Verification items for the finished model (mm, model axes). A direction names the side the tool comes from. Round coordinates to 2 decimals unless told otherwise and drop trailing zeros. Write each loop counter-clockwise with the first axis right and the second up, starting at its lowest first coordinate (ties: lowest second). Pieces come first, ordered by that corner, then holes. Notation, with made-up numbers: M -33.75,48 L 9.25,48 A35 cw 9.25,82 Z; hole C 71,-8.5 d10. An arc over 180 degrees is marked long. Answer in a Markdown table with one row per item. Add a question column.
1. Set-up check for faces 5 (the flat face through (25, 75, -37.5)), 6 (the flat face through (25, 75, -46.015)), 7 (the cylindrical face through (5.505, 6.451, -42.813)): record each of +Z, -Z, +X, -X, +Y, -Y from which the full face is reachable in a straight line by a thin tool's end or side.
2. Material ranges on probe 1 along X at (y, z) = (75, -40.5); probe 2 along Y at (x, z) = (35, -39); probe 3 along Z at (x, y) = (5, 7), recorded low to high.
3. Go/stop test with flat-tipped pins: pin 1 Ø2 at (x, y) = (16.5, 30) entering from -Z; pin 2 Ø2.5 at (x, y) = (35, 75) entering from -Z; pin 3 Ø4 at (x, y) = (42.5, 54) entering from -Z; pin 4 Ø1 at (x, z) = (43.5, -19.5) entering from -Y. Record where each tip stops, or that it passes through.
4. Sectioned sample at A-A on y = 75. Record the cut outline in (x, z).
5. Draft check along X on faces 1 (the flat face through (50, 42, -19)), 2 (the flat face through (25, 0, -44)), 3 (the flat face through (42.76, 1.48, -41.69)), 4 (the flat face through (2.669, 1, -6)). Enter one of: pulls with the +X half, pulls with the -X half, needs draft (parallel to the pull), parting line crosses it, or undercut.
6. Sectioned sample at B-B on z = -44.3. Record the cut outline in (x, y).
7. Sectioned sample at C-C on x = 34. Count the separate pieces of the cut face and the enclosed holes in it, plus the area to 3 significant figures.
Autodesk Inventor part; units mm, degrees
ref_plane "YZ Plane" through (0, 0, 0) normal (1, 0, 0) x (0, 1, 0)
ref_plane "XZ Plane" through (0, 0, 0) normal (0, 1, 0) x (-1, 0, 0)
ref_plane "XY Plane" through (0, 0, 0) normal (0, 0, 1) x (1, 0, 0)
sketch "Sketch1" plane through (0, 0, 0) normal (1, 0, 0) x (0, 1, 0)
  ellipse E0 centre (0, -25) end of major axis (45, -25) minor radius 12.5 (0, -37.5) -> (0, -12.5) ccw
  ellipse E1 centre (0, -25) end of major axis (120, -25) minor radius 25 (0, -50) -> (0, 0) ccw
  line L0 (65, -3.9852) -> (65, -46.0148)
  line L1 (0, -37.5) -> (0, -50)
  line L2 (0, -12.5) -> (0, 0)
  point P0 (0, -43.75)
  point P1 (0, -6.25)
  dimension "d23" = 45
  dimension "d25" = 120
  dimension "d18" = 50
  dimension "d22" = 25
  dimension "d24" = 65
extrude "Extrusion1" add sketch "Sketch1" along normal blind 50 contours E0 L2 E1 L0 L1
sketch "Sketch3" plane through (0, 65, -3.9852) normal (0, 1, 0) x (1, 0, 0)
  line L0 (0, 42.0297) -> (0, 0)
  line L1 (0, 0) -> (50, 0)
  line L2 (50, 42.0297) -> (50, 0)
  line L3 (0, 42.0297) -> (50, 42.0297)
  line L4 (0, 33.5148) -> (0, 8.5148)
  line L5 (50, 0) -> (0, 0)
  line L6 (0, 0) -> (0, 8.5148)
  line L7 (0, 8.5148) -> (50, 8.5148)
  line L8 (50, 8.5148) -> (50, 0)
  line L9 (0, 42.0297) -> (50, 42.0297)
  line L10 (50, 42.0297) -> (50, 33.5148)
  line L11 (50, 33.5148) -> (0, 33.5148)
  line L12 (0, 33.5148) -> (0, 42.0297)
  point P0 (0, -3.9852)
  point P1 (0, 33.5148)
  dimension "d26" = 25
  dimension "d27" = 8.5148
  dimension "d28" = 8.5148
extrude "Extrusion3" add sketch "Sketch3" along normal blind 20 contours L3 L2 L11 L0 | L7 L2 L1 L0
sketch "Sketch4" plane through (50, 65, -46.0148) normal (0, 0, -1) x (-1, 0, 0)
  line L0 (50, 0) -> (0, 0)
  line L1 (50, 0) -> (50, 20)
  line L2 (0, 20) -> (50, 20)
  line L3 (0, 0) -> (0, 20)
  line L4 (0, 0) -> (0, 20)
  line L5 (0, 10) -> (50, 10)
  circle A0 centre (15, 10) radius 2.25
  circle A1 centre (35, 10) radius 2.25
  point P0 (50, -65)
  dimension "d31" = 4.5
  dimension "d32" = 4.5
  dimension "d33" = 20
  dimension "d34" = 15
  dimension "d35" = 15
extrude "Extrusion4" cut sketch "Sketch4" against normal through all contours A1 L5 | L5 A1 | A0 L5 | L5 A0
sketch "Sketch5" plane through (0, 0, -12.5) normal (0, -1, 0) x (1, 0, 0)
  line L0 (0, 12.5) -> (0, 0)
  line L1 (0, 0) -> (50, 0)
  line L2 (50, 12.5) -> (50, 0)
  line L3 (0, 12.5) -> (50, 12.5)
  line L4 (0, -25) -> (0, -37.5)
  line L5 (0, -37.5) -> (50, -37.5)
  line L6 (50, -25) -> (50, -37.5)
  line L7 (0, -25) -> (50, -25)
  line L8 (50, 8.5148) -> (50, 12.5)
  line L9 (0, -25) -> (0, -37.5)
  line L10 (50, 12.5) -> (0, -37.5)
  line L11 (5.7, 6.8) -> (44.3, 6.8)
  line L12 (44.3, 6.8) -> (44.3, -31.8)
  line L13 (44.3, -31.8) -> (5.7, -31.8)
  line L14 (5.7, -31.8) -> (5.7, 6.8)
  line L15 (5.7, 6.8) -> (44.3, -31.8) construction
  line L16 (44.3, 6.8) -> (5.7, -31.8) construction
  line L17 (44.3, 3.3) -> (41.2689, 5.05)
  line L18 (41.2689, 5.05) -> (41.2689, 8.55)
  line L19 (41.2689, 8.55) -> (44.3, 10.3)
  line L20 (44.3, 10.3) -> (47.3311, 8.55)
  line L21 (47.3311, 8.55) -> (47.3311, 5.05)
  line L22 (47.3311, 5.05) -> (44.3, 3.3)
  line L23 (41.2689, -33.55) -> (41.2689, -30.05)
  line L24 (41.2689, -30.05) -> (44.3, -28.3)
  line L25 (44.3, -28.3) -> (47.3311, -30.05)
  line L26 (47.3311, -30.05) -> (47.3311, -33.55)
  line L27 (47.3311, -33.55) -> (44.3, -35.3)
  line L28 (44.3, -35.3) -> (41.2689, -33.55)
  line L29 (8.7311, -30.05) -> (8.7311, -33.55)
  line L30 (8.7311, -33.55) -> (5.7, -35.3)
  line L31 (5.7, -35.3) -> (2.6689, -33.55)
  line L32 (2.6689, -33.55) -> (2.6689, -30.05)
  line L33 (2.6689, -30.05) -> (5.7, -28.3)
  line L34 (5.7, -28.3) -> (8.7311, -30.05)
  line L35 (8.7311, 8.55) -> (8.7311, 5.05)
  line L36 (8.7311, 5.05) -> (5.7, 3.3)
  line L37 (5.7, 3.3) -> (2.6689, 5.05)
  line L38 (2.6689, 5.05) -> (2.6689, 8.55)
  line L39 (2.6689, 8.55) -> (5.7, 10.3)
  line L40 (5.7, 10.3) -> (8.7311, 8.55)
  point P0 (25, -12.5)
  dimension "d38" = 38.6
  dimension "d39" = 38.6
  dimension "d40" = 7
  dimension "d41" = 7
  dimension "d42" = 7
  dimension "d43" = 7
extrude "Extrusion5" cut sketch "Sketch5" against normal blind 3 contours L20 L21 L22 L12 L10 | L10 L11 L18 L19 L20 | L37 L38 L39 L40 L35 L11 L14 | L14 L11 L35 L36 | L12 L17 L10 | L10 L17 L18 L11 | L34 L10 L14 | L14 L10 L31 L32 L33 | L34 L29 L13 L10 | L13 L29 L30 L31 L10 | L25 L26 L27 L28 L23 L13 L12 | L12 L13 L23 L24
sketch "Sketch6" plane through (0, 0, -12.5) normal (0, -1, 0) x (1, 0, 0)
  line L0 (44.3, 10.3) -> (47.3311, 8.55)
  line L1 (41.2689, 8.55) -> (44.3, 10.3)
  line L2 (41.2689, 5.05) -> (41.2689, 8.55)
  line L3 (44.3, 3.3) -> (41.2689, 5.05)
  line L4 (47.3311, 5.05) -> (44.3, 3.3)
  line L5 (47.3311, 8.55) -> (47.3311, 5.05)
  line L6 (47.3311, -33.55) -> (44.3, -35.3)
  line L7 (47.3311, -30.05) -> (47.3311, -33.55)
  line L8 (44.3, -28.3) -> (47.3311, -30.05)
  line L9 (41.2689, -30.05) -> (44.3, -28.3)
  line L10 (41.2689, -33.55) -> (41.2689, -30.05)
  line L11 (44.3, -35.3) -> (41.2689, -33.55)
  line L12 (5.7, -35.3) -> (2.6689, -33.55)
  line L13 (8.7311, -33.55) -> (5.7, -35.3)
  line L14 (8.7311, -30.05) -> (8.7311, -33.55)
  line L15 (5.7, -28.3) -> (8.7311, -30.05)
  line L16 (2.6689, -30.05) -> (5.7, -28.3)
  line L17 (2.6689, -33.55) -> (2.6689, -30.05)
  line L18 (2.6689, 8.55) -> (5.7, 10.3)
  line L19 (2.6689, 5.05) -> (2.6689, 8.55)
  line L20 (5.7, 3.3) -> (2.6689, 5.05)
  line L21 (8.7311, 5.05) -> (5.7, 3.3)
  line L22 (8.7311, 8.55) -> (8.7311, 5.05)
  line L23 (5.7, 10.3) -> (8.7311, 8.55)
  line L24 (8.7311, 8.55) -> (2.6689, 5.05)
  circle A0 centre (5.7, 6.8) radius 1.5
  line L25 (2.6689, -30.05) -> (8.7311, -33.55)
  line L26 (47.3311, -33.55) -> (44.3, -35.3)
  line L27 (41.2689, -30.05) -> (47.3311, -33.55)
  line L28 (41.2689, 5.05) -> (41.2689, 8.55)
  line L29 (47.3311, 5.05) -> (44.3, 3.3)
  line L30 (41.2689, 8.55) -> (47.3311, 5.05)
  circle A1 centre (44.3, 6.8) radius 1.5
  circle A2 centre (44.3, -31.8) radius 1.5
  circle A3 centre (5.7, -31.8) radius 1.5
  point P0 (0, 12.5)
  dimension "d46" = 3
  dimension "d47" = 3
  dimension "d48" = 3
  dimension "d49" = 3
extrude "Extrusion6" cut sketch "Sketch6" against normal blind 10 contours A1 L30 | L30 A1 | A2 L27 | L27 A2 | A3 L25 | L25 A3 | A0 L24 | L24 A0
equation "\"d27\" = d28"
properties part number "Arch" material "ABS Plastic"
Geometry check:
| question | item | result |
|---|---|---|
| 1 | face 5 | +X, -X, +Y |
| 1 | face 6 | -Z, +X, -X, +Y |
| 1 | face 7 | -Y |
| 2 | probe 1 | x = 0 to 12.75, 17.25 to 32.75, 37.25 to 50 |
| 2 | probe 2 | y = 0 to 72.75, 77.25 to 85 |
| 2 | probe 3 | z = -49.96 to -45.63, -42.97 to -37.35, -12.65 to -7.03, -4.37 to -0.04 |
| 3 | pin 1 | stops at z = -49.26 |
| 3 | pin 2 | passes through |
| 3 | pin 3 | stops at z = -47.53 |
| 3 | pin 4 | stops at y = 39.48 |
| 4 | outline | M 0,-46.01 L 12.75,-46.01 L 12.75,-37.5 L 0,-37.5 Z; M 0,-12.5 L 12.75,-12.5 L 12.75,-3.99 L 0,-3.99 Z; M 17.25,-46.01 L 32.75,-46.01 L 32.75,-37.5 L 17.25,-37.5 Z; M 17.25,-12.5 L 32.75,-12.5 L 32.75,-3.99 L 17.25,-3.99 Z; M 37.25,-46.01 L 50,-46.01 L 50,-37.5 L 37.25,-37.5 Z; M 37.25,-12.5 L 50,-12.5 L 50,-3.99 L 37.25,-3.99 Z |
| 5 | face 1 | pulls with the +X half |
| 5 | face 2 | needs draft |
| 5 | face 3 | undercut |
| 5 | face 4 | undercut |
| 6 | outline | M 0,0 L 2.67,0 L 2.67,3 L 4.2,3 L 4.2,10 L 7.2,10 L 7.2,3 L 8.73,3 L 8.73,0 L 41.27,0 L 41.27,3 L 42.8,3 L 42.8,10 L 45.8,10 L 45.8,3 L 47.33,3 L 47.33,0 L 50,0 L 50,85 L 0,85 Z; hole C 15,75 d4.5; hole C 35,75 d4.5 |
| 7 | separate pieces | 3 |
| 7 | enclosed holes | 0 |
| 7 | area | 2,470 mm2 |
